```python
from build123d import *

# Parameters (mm, degrees)
F0_W     = 100
F0_H     = 100
F1_DEPTH = 10
F3_DEPTH = 28
F4_R     = 2
F5_DEPTH = 305
F6_R     = 2
F7_DEPTH = 305
F8_W     = 14
F8_H     = 24
F8_H_2   = 14
F9_DEPTH = 305
F10_SIZE = 4.99999


# Not quite as in the source:
# - a fillet or chamfer is up to 0.001 mm smaller than in the source, because OpenCascade refuses the exact size


with BuildPart() as f1:
    # F0 (on Top) → F1 (new body)
    with BuildSketch(Plane.XY):
        with Locations((-5.6718036532, 2.052295208)):
            Rectangle(F0_W, F0_H)
    extrude(amount=F1_DEPTH)

    # F2 (on Top) → F3 (cut)
    with BuildSketch(Plane.XY):
        Polygon((-8.8692104674, -10.7118982853), (1.3029770516, -13.8459347822), (10.7118982853, -8.8692104674), (13.8459347822, 1.3029770516), (8.8692104674, 10.7118982853), (-1.3029770516, 13.8459347822), (-10.7118982853, 8.8692104674), (-13.8459347822, -1.3029770516), align=None)
    extrude(amount=F3_DEPTH, mode=Mode.SUBTRACT)

    # F4 (on Top) → F5 (join)
    with BuildSketch(Plane.XY):
        with Locations((24.3281963468, -27.947704792)):
            Circle(F4_R)
    extrude(amount=-F5_DEPTH)

    # F6 (on Top) → F7 (join)
    with BuildSketch(Plane.XY):
        with Locations((-35.6718036532, 32.052295208)):
            Circle(F6_R)
    extrude(amount=-F7_DEPTH)

    # F8 (on Top) → F9 (join)
    with BuildSketch(Plane.XY):
        with Locations((-42.6718036532, -29.947704792)):
            Rectangle(F8_W, F8_H)
        with Locations((31.3281963468, 39.052295208)):
            Rectangle(F8_W, F8_H_2)
    extrude(amount=-F9_DEPTH)

    # F10 (size 5 in the source; OpenCascade refuses exactly that, so slightly less here)
    f10_edges = [f1.edges().sort_by_distance(p)[0] for p in [
        (-55.671804, 2.052295, 10),
        (-5.671804, -47.947705, 10),
        (-5.671804, 52.052295, 0),
        (44.328196, 2.052295, 10),
    ]]
    chamfer(f10_edges, length=F10_SIZE)


solid = f1.part
```
CAD build for the part. Positions are in the model's coordinates, mm. A direction names the side the tool comes from. Coordinates: 2 decimals unless noted, no trailing zeros. Order: outer loops, then holes, each group sorted by start corner. A loop starts at its lowest first (then second) coordinate and runs counter-clockwise, first axis right, second up. Notation, with made-up numbers: (15.5, 18.25) -> (54.5, 18.25) arc R23 cw to (54.5, 57.25) -> close; hole circle Ø9 at (-3, 32.25). An arc over 180 degrees is marked (long way). Use one line per item in the form item = value. Start each with the question number.
1) Tool access for faces 1 (the flat face through (-49.672, -30, -150)), 2 (the flat face through (-43, -41.948, -150)), 3 (the flat face through (12.26, -3.85, 4.93)), 4 (the flat face through (31, 46.052, -150)): list every direction of +Z, -Z, +X, -X, +Y, -Y with a clear straight run to the whole face (end or side of a thin tool).
2) Band-saw the part on A-A on z = -137. Give the cut face in (x, y), then the cut area to 3 significant figures.
3) Band-saw the part on B-B on y = 43. Give the cut face in (x, z).
4) Band-saw the part on D-D on x = 30. Give the cut face in (y, z), then the cut area to 4 significant figures.
5) Drop flat-ended pins along their axis: pin 1 (7 mm diameter, centred on y = 39, z = -176.5, fed in from -X); pin 2 (12 mm diameter, centred on x = -28, z = -172, fed in from +Y); pin 3 (11 mm diameter, centred on y = 36.5, z = -190, fed in from +X). Give the stop position or say it passes through.
6) Drill centre lines: L1, parallel to Z at x = -35, y = -23; L2, parallel to X at y = 42.5, z = -246; L3, parallel to Y at x = -44, z = -173. Where is each one in solid material? Low to high. Write a range as [from, to].
7) Band-saw the part on C-C on x = 5.5. Give the cut face in (y, z).
Entries:
q1.face_1 = -Z, -X, +Y, -Y
q1.face_2 = -Z, +X, -X, -Y
q1.face_3 = +Z, -Z
q1.face_4 = -Z, +X, -X, +Y
q2.outline = (-49.67, -41.95) -> (-35.67, -41.95) -> (-35.67, -17.95) -> (-49.67, -17.95) -> close; circle Ø4 at (-35.67, 32.05); circle Ø4 at (24.33, -27.95); (24.33, 32.05) -> (38.33, 32.05) -> (38.33, 46.05) -> (24.33, 46.05) -> close
q2.area = 557 mm2
q3.outline = (-55.67, 0) -> (24.33, 0) -> (24.33, -305) -> (38.33, -305) -> (38.33, 0) -> (44.33, 0) -> (44.33, 5) -> (39.33, 10) -> (-50.67, 10) -> (-55.67, 5) -> close
q4.outline = (-47.95, 0) -> (32.05, 0) -> (32.05, -305) -> (46.05, -305) -> (46.05, 0) -> (47.05, 0) -> (52.05, 5) -> (52.05, 10) -> (-42.95, 10) -> (-47.95, 5) -> close
q4.area = 5,245 mm2
q5.pin_1 = 24.33
q5.pin_2 = 33.15
q5.pin_3 = 38.33
q6.L1 = [0, 10]
q6.L2 = [24.33, 38.33]
q6.L3 = [-41.95, -17.95]
q7.outline = (-47.95, 0) -> (-11.63, 0) -> (-11.63, 10) -> (-42.95, 10) -> (-47.95, 5) -> close; (11.75, 0) -> (47.05, 0) -> (52.05, 5) -> (52.05, 10) -> (11.75, 10) -> close
